Here's how the part is built. I have some questions about the finished solid (model axes, mm). Face numbers are marked on the shaded views. A direction names the side the tool comes from. Round coordinates to 2 decimals unless told otherwise and drop trailing zeros. Order: outer loops, then holes, each group sorted by start corner. A loop starts at its lowest first (then second) coordinate and runs counter-clockwise, first axis right, second up. Notation, with made-up numbers: M -31,87.25 L 10,87.25 A20 cw 10,113.25 Z; hole C 30,15.25 d3. An arc over 180 degrees is marked long. Answer as CSV lines item,"result". Start each with the question number.
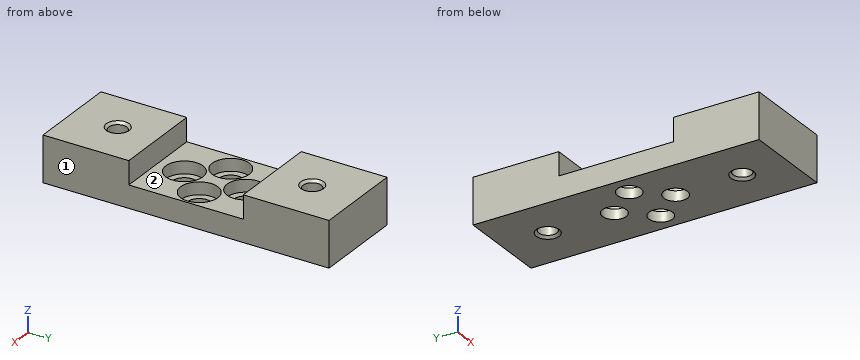
Autodesk Inventor part; units mm, degrees
ref_plane "screw1_XY" through (-6.9088, 0, -3.429) normal (0, 0, 1) x (1, 0, 0)
ref_plane "screw1_YZ" through (-6.9088, 0, -3.429) normal (1, 0, 0) x (0, 1, 0)
ref_plane "screw1_ZX" through (-6.9088, 0, -3.429) normal (0, 1, 0) x (0, 0, 1)
sketch "Sketch_1" plane through (0, 0, 0) normal (1, 0, 0) x (0, 1, 0)
  line L0 (-15.8877, 6.477) -> (-39.6875, 6.477)
  line L1 (-39.6875, 6.477) -> (-39.6875, -6.223)
  line L2 (-39.6875, -6.223) -> (39.6875, -6.223)
  line L3 (39.6875, -6.223) -> (39.6875, 6.477)
  line L4 (39.6875, 6.477) -> (15.8877, 6.477)
  line L5 (15.8877, 6.477) -> (15.8877, 0)
  line L6 (15.8877, 0) -> (-15.8877, 0)
  line L7 (-15.8877, 0) -> (-15.8877, 6.477)
extrude "Extrusion1" add sketch "Sketch_1" along normal mid plane 25.4
sketch "Sketch_2" plane through (0, 0, 0) normal (1, 0, 0) x (0, 1, 0)
  line L0 (26.9875, -6.223) -> (26.9875, 6.477)
  line L1 (26.9875, 6.477) -> (30.1625, 6.477)
  line L2 (30.1625, 6.477) -> (29.4754, 5.7899)
  line L3 (29.4754, 5.7899) -> (29.4754, -5.5359)
  line L4 (29.4754, -5.5359) -> (30.1625, -6.223)
  line L5 (30.1625, -6.223) -> (26.9875, -6.223)
  line L6 (26.9875, -6.223) -> (26.9875, 6.477)
revolve "Revolution1" cut sketch "Sketch_2" angle 360 about axis through (0, 26.9875, -6.223) along (0, 0, -1)
thread "Thread1"
sketch "Sketch_3" plane through (0, 0, 0) normal (1, 0, 0) x (0, 1, 0)
  line L0 (-26.9875, -6.223) -> (-26.9875, 6.477)
  line L1 (-26.9875, 6.477) -> (-23.8125, 6.477)
  line L2 (-23.8125, 6.477) -> (-24.4996, 5.7899)
  line L3 (-24.4996, 5.7899) -> (-24.4996, -5.5359)
  line L4 (-24.4996, -5.5359) -> (-23.8125, -6.223)
  line L5 (-23.8125, -6.223) -> (-26.9875, -6.223)
  line L6 (-26.9875, -6.223) -> (-26.9875, 6.477)
revolve "Revolution2" cut sketch "Sketch_3" angle 360 about axis through (0, -26.9875, -6.223) along (0, 0, -1)
thread "Thread2"
sketch "Sketch4" plane through (-12.7, -15.8877, 0) normal (0, 0, 1) x (1, 0, 0)
  point P0 (5.7912, 15.8877)
hole "Hole1" at (-6.9088, 0, 0) direction (0, 0, -1) diameter 6.5278 depth 6.223 counterbore diameter 10.3124 counterbore depth 3.429
pattern_linear "Rectangular Pattern1" count 2 spacing 10.9507 along (0.6309, 0.7759, 0) count 2 spacing 10.9507 along (0.6309, -0.7759, 0) of "Hole1"
ref_plane "screw1_XY" through (-6.9088, 0, -3.429) normal (0, 0, 1) x (1, 0, 0)
ref_plane "screw1_YZ" through (-6.9088, 0, -3.429) normal (1, 0, 0) x (0, 1, 0)
ref_plane "screw1_ZX" through (-6.9088, 0, -3.429) normal (0, 1, 0) x (0, 0, 1)
ref_plane "screw1_1_XY" through (0, 8.4963, -3.429) normal (0, 0, 1) x (1, 0, 0)
ref_plane "screw1_1_YZ" through (0, 8.4963, -3.429) normal (1, 0, 0) x (0, 1, 0)
ref_plane "screw1_1_ZX" through (0, 8.4963, -3.429) normal (0, 1, 0) x (0, 0, 1)
ref_plane "screw2_XY" through (6.9088, 0, -3.429) normal (0, 0, 1) x (1, 0, 0)
ref_plane "screw2_YZ" through (6.9088, 0, -3.429) normal (1, 0, 0) x (0, 1, 0)
ref_plane "screw2_ZX" through (6.9088, 0, -3.429) normal (0, 1, 0) x (0, 0, 1)
ref_plane "screw2_1_XY" through (0, -8.4963, -3.429) normal (0, 0, 1) x (1, 0, 0)
ref_plane "screw2_1_YZ" through (0, -8.4963, -3.429) normal (1, 0, 0) x (0, 1, 0)
ref_plane "screw2_1_ZX" through (0, -8.4963, -3.429) normal (0, 1, 0) x (0, 0, 1)
ref_plane "to_dummy_XY" through (0, 0, -6.223) normal (0, 0, 1) x (1, 0, 0)
ref_plane "to_dummy_YZ" through (0, 0, -6.223) normal (1, 0, 0) x (0, 1, 0)
ref_plane "to_dummy_ZX" through (0, 0, -6.223) normal (0, 1, 0) x (0, 0, 1)
ref_plane "to_screw1_XY" through (0, 26.9875, 6.477) normal (0, 0, 1) x (1, 0, 0)
ref_plane "to_screw1_YZ" through (0, 26.9875, 6.477) normal (1, 0, 0) x (0, 1, 0)
ref_plane "to_screw1_ZX" through (0, 26.9875, 6.477) normal (0, 1, 0) x (0, 0, 1)
ref_plane "to_screw2_XY" through (0, -26.9875, 6.477) normal (0, 0, 1) x (1, 0, 0)
ref_plane "to_screw2_YZ" through (0, -26.9875, 6.477) normal (1, 0, 0) x (0, 1, 0)
ref_plane "to_screw2_ZX" through (0, -26.9875, 6.477) normal (0, 1, 0) x (0, 0, 1)
properties part number "2750-1_b"
Item 1: If we section it at C-C on x = 9.25: Please give me the cut outline in (y, z), and give its area (3 significant figures).
Item 2: For P1, Ø5, axis at x = 2.5, y = 7.5, coming from the +Z side; P2, Ø8, axis at x = -6, y = 0.5, coming from the +Z side; P3, Ø6, axis at x = -6.91, y = 0, coming from the +Z side, each with a flat end and sliding along its axis, tell me the tip position at first contact or that it passes through.
Item 3: Which directions (+Z, -Z, +X, -X, +Y, -Y) give clear straight access to the entire face, cutting with the end or side of a thin tool? Please do the marked faces 1 and 2.
Item 4: If I drill on line 1 along X through (y, z) = (0, -4.3); line 2 along Y through (x, z) = (8.75, 4); line 3 along X through (y, z) = (0, -1.8) (3 decimals), over which ranges is the centre line in solid material (lowest first)?
Item 5: If we section it at A-A on z = 2: Please give me the cut outline in (x, y).
Item 6: If we section it at D-D on y = 9.5: Please give me the cut outline in (x, z), and give its area (3 significant figures).
Item 7: If we section it at B-B on y = 0: Please give me the cut outline in (x, z) (1 decimal), and give its area (3 significant figures).
Geometry says:
1,outline,"M -39.69,-6.22 L -2.27,-6.22 L -2.27,-3.43 L -4.59,-3.43 L -4.59,0 L -15.89,0 L -15.89,6.48 L -39.69,6.48 Z; M 2.27,-6.22 L 39.69,-6.22 L 39.69,6.48 L 15.89,6.48 L 15.89,0 L 4.59,0 L 4.59,-3.43 L 2.27,-3.43 Z"
1,area,"758 mm²"
2,P1,"z = 0"
2,P2,"z = -3.43"
2,P3,"through"
3,face 1,"+Z, -Z, +X, +Y, -Y"
3,face 2,"+Z, +X, -X"
4,line 1,"-12.7 to -10.17, -3.64 to 3.64, 10.17 to 12.7"
4,line 2,"-39.69 to -15.89, 15.89 to 39.69"
4,line 3,"-12.7 to -12.065, -1.753 to 1.752, 12.065 to 12.7"
5,outline,"M -12.7,-39.69 L 12.7,-39.69 L 12.7,-15.89 L -12.7,-15.89 Z; M -12.7,15.89 L 12.7,15.89 L 12.7,39.69 L -12.7,39.69 Z; hole C 0,-26.99 d4.98; hole C 0,26.99 d4.98"
6,outline,"M -12.7,-6.22 L -3.11,-6.22 L -3.11,-3.43 L -5.06,-3.43 L -5.06,0 L -12.7,0 Z; M 3.11,-6.22 L 12.7,-6.22 L 12.7,0 L 5.06,0 L 5.06,-3.43 L 3.11,-3.43 Z"
6,area,"106 mm²"
7,outline,"M -12.7,-6.2 L -10.2,-6.2 L -10.2,-3.4 L -12.1,-3.4 L -12.1,0 L -12.7,0 Z; M -3.6,-6.2 L 3.6,-6.2 L 3.6,-3.4 L 1.8,-3.4 L 1.8,0 L -1.8,0 L -1.8,-3.4 L -3.6,-3.4 Z; M 10.2,-6.2 L 12.7,-6.2 L 12.7,0 L 12.1,0 L 12.1,-3.4 L 10.2,-3.4 Z"
7,area,"50.9 mm²"
